CAD build for the part. Positions are in the model's coordinates, mm. A direction names the side the tool comes from. Round coordinates to 2 decimals unless told otherwise and drop trailing zeros. Order: outer loops, then holes, each group sorted by start corner. A loop starts at its lowest first (then second) coordinate and runs counter-clockwise, first axis right, second up. Notation, with made-up numbers: (-27.75, -18) -> (22.25, -18) arc R18 cw to (22.25, 8) -> close; hole circle Ø2 at (37.25, 22). An arc over 180 degrees is marked (long way). Return JSON: item names as keys, results as strings. Group by question number.
Q1. Cut at C-C (x = -19). Write the cut outline in (y, z), then the cut area to 3 significant figures.
Q2. Flat gauge pins, fed straight in: pin 1 (2.5 mm diameter, centred on y = 18.5, z = 6, fed in from +X); pin 2 (2.5 mm diameter, centred on x = -25.5, z = 7, fed in from +Y); pin 3 (4 mm diameter, centred on y = 20, z = 4.5, fed in from -X). Where does each tip first touch, or does it go through?
Q3. Cut at D-D (z = 5.5). Write the cut outline in (x, y).
Q4. Which spindle directions (+Z, -Z, +X, -X, +Y, -Y) get a long thin tool onto all of the face, cutting with end or side? Do faces 1 (the flat face through (-22, 19, 5)), 2 (the cylindrical face through (-23.945, -3.218, 4.93)), 3 (the flat face through (26, 15, 5)). Say none if no direction does.
Q5. Cut at B-B (y = -3). Write the cut outline in (x, z), then the cut area to 3 significant figures.
Q6. Cut at A-A (x = 0). Write the cut outline in (y, z).
Q7. Mould opens along Y. For faces 4 (the flat face through (0, 4, 0)), 5 (the flat face through (0, -15, 5)), 6 (the cylindrical face through (14.055, -3.218, 4.93)), 7 (the cylindrical face through (-3.648, -6.345, 4.93)) say: +Y half, -Y half, draft (parallel to the pull), parting line (faces both ways), or undercut.
Q8. Probe line 1 along Y through (x, z) = (0, 7.75); line 2 along Y through (x, z) = (2, 4.5); line 3 along X through (y, z) = (8.5, 5.5). List the from-to ranges inside material, lowest first.
from build123d import *

# Parameters (mm, degrees)
F0_R     = 2.9
F0_W     = 44
F0_H     = 8
F1_DEPTH = 10


with BuildPart() as f1:
    # F0 (on Top) → F1 (new body)
    with BuildSketch(Plane.XY):
        with BuildLine():
            Line((23.95, -3), (30, -3))
            Line((30, -3), (30, 15))
            Line((30, 15), (22, 15))
            Line((22, 15), (-22, 15))
            Line((-22, 15), (-30, 15))
            Line((-30, 15), (-30, -3))
            Line((-30, -3), (-23.95, -3))
            ThreePointArc((-23.95, -3), (-19, 1.95), (-14.05, -3))
            Line((-14.05, -3), (-4.95, -3))
            ThreePointArc((-4.95, -3), (0, 1.95), (4.95, -3))
            Line((4.95, -3), (14.05, -3))
            ThreePointArc((14.05, -3), (19, 1.95), (23.95, -3))
        make_face()
        with Locations((0, 8.284595)):
            Circle(F0_R, mode=Mode.SUBTRACT)
        with BuildLine():
            Line((-30, -15), (30, -15))
            Line((30, -15), (30, -3))
            Line((30, -3), (23.95, -3))
            ThreePointArc((23.95, -3), (19, -7.95), (14.05, -3))
            Line((14.05, -3), (4.95, -3))
            ThreePointArc((4.95, -3), (0, -7.95), (-4.95, -3))
            Line((-4.95, -3), (-14.05, -3))
            ThreePointArc((-14.05, -3), (-19, -7.95), (-23.95, -3))
            Line((-23.95, -3), (-30, -3))
            Line((-30, -3), (-30, -15))
        make_face()
        with Locations((0, 19)):
            Rectangle(F0_W, F0_H)
    extrude(amount=F1_DEPTH)


solid = f1.part
Solution:
{
 "1": {"outline": "(-15, 0) -> (-7.95, 0) -> (-7.95, 10) -> (-15, 10) -> close; (1.95, 0) -> (23, 0) -> (23, 10) -> (1.95, 10) -> close", "area": "281 mm²"},
 "2": {"pin 1": "stops at x = 22", "pin 2": "stops at y = 15", "pin 3": "stops at x = -22"},
 "3": {"outline": "(-30, -15) -> (30, -15) -> (30, 15) -> (22, 15) -> (22, 23) -> (-22, 23) -> (-22, 15) -> (-30, 15) -> close; hole circle Ø9.9 at (-19, -3); hole circle Ø9.9 at (0, -3); hole circle Ø5.8 at (0, 8.28); hole circle Ø9.9 at (19, -3)"},
 "4": {"face 1": "+Z, -Z, -X, +Y", "face 2": "+Z, -Z", "face 3": "+Z, -Z, +X, +Y"},
 "5": {"outline": "(-30, 0) -> (-23.95, 0) -> (-23.95, 10) -> (-30, 10) -> close; (-14.05, 0) -> (-4.95, 0) -> (-4.95, 10) -> (-14.05, 10) -> close; (4.95, 0) -> (14.05, 0) -> (14.05, 10) -> (4.95, 10) -> close; (23.95, 0) -> (30, 0) -> (30, 10) -> (23.95, 10) -> close", "area": "303 mm²"},
 "6": {"outline": "(-15, 0) -> (-7.95, 0) -> (-7.95, 10) -> (-15, 10) -> close; (1.95, 0) -> (5.38, 0) -> (5.38, 10) -> (1.95, 10) -> close; (11.18, 0) -> (23, 0) -> (23, 10) -> (11.18, 10) -> close"},
 "7": {"face 4": "draft", "face 5": "-Y half", "face 6": "undercut", "face 7": "undercut"},
 "8": {"line 1": "y = -15 to -7.95, 1.95 to 5.38, 11.18 to 23", "line 2": "y = -15 to -7.53, 1.53 to 6.18, 10.38 to 23", "line 3": "x = -30 to -2.89, 2.89 to 30"}
}
